Input: part model. Units: mm. Frame: model coordinates. Face numbers are marked on the shaded views. A direction names the side the tool comes from. Round coordinates to 2 decimals unless told otherwise and drop trailing zeros. Order: outer loops, then holes, each group sorted by start corner. A loop starts at its lowest first (then second) coordinate and runs counter-clockwise, first axis right, second up. Notation, with made-up numbers: (13, 19) -> (20, 19) arc R22 cw to (20, 56) -> close; hole circle Ø8 at (13, -39). An arc over 180 degrees is marked (long way). Use a Markdown table: item, result.
from build123d import *

# Parameters (mm, degrees)
BOSS_EXTRUDE1_DEPTH         = 2
SKETCH5_R                   = 4
SKETCH5_R_2                 = 1.998542518
BOSS_EXTRUDE2_DEPTH         = 3
SKETCH8_R                   = 1.5
CUT_EXTRUDE2_DEPTH          = 6
SKETCH9_R                   = 3.6
SKETCH9_R_2                 = 3
BOSS_EXTRUDE3_DEPTH         = 0.85
SKETCH10_R                  = 0.75
CUT_EXTRUDE3_DEPTH          = 2
LPATTERN1_COUNT             = 4
LPATTERN1_PITCH             = 3.5
CIRPATTERN1_COUNT           = 4
CIRPATTERN1_COPY_1_SKETCH_R = 0.75
CIRPATTERN1_COPY_1_DEPTH    = 2
CIRPATTERN1_COPY_2_SKETCH_R = 0.75
CIRPATTERN1_COPY_2_DEPTH    = 2
CIRPATTERN1_COPY_3_SKETCH_R = 0.75
CIRPATTERN1_COPY_3_DEPTH    = 2
CIRPATTERN1_COPY_4_SKETCH_R = 0.75
CIRPATTERN1_COPY_4_DEPTH    = 2
CIRPATTERN1_COPY_5_SKETCH_R = 0.75
CIRPATTERN1_COPY_5_DEPTH    = 2
CIRPATTERN1_COPY_6_SKETCH_R = 0.75
CIRPATTERN1_COPY_6_DEPTH    = 2
CIRPATTERN1_COPY_7_SKETCH_R = 0.75
CIRPATTERN1_COPY_7_DEPTH    = 2
CIRPATTERN1_COPY_8_SKETCH_R = 0.75
CIRPATTERN1_COPY_8_DEPTH    = 2
CIRPATTERN1_COPY_9_SKETCH_R = 0.75
CIRPATTERN1_COPY_9_DEPTH    = 2


with BuildPart() as part:
    # Sketch1 → Boss-Extrude1 (new body)
    with BuildSketch(Plane(origin=(0, 0, 0), x_dir=(1, 0, 0), z_dir=(0, 1, 0))):
        with BuildLine():
            Line((11.195476756, 1.969359322), (4.786657556, -6.592741724))
            ThreePointArc((4.786657556, -6.592741724), (3.929987754, -8.118293207), (4.786657556, -9.643844691))
            Line((4.786657556, -9.643844691), (11.195476756, -18.205945736))
            ThreePointArc((11.195476756, -18.205945736), (10.933214648, -21.871520101), (7.267640283, -22.133782209))
            Line((7.267640283, -22.133782209), (-1.294460762, -15.724963009))
            ThreePointArc((-1.294460762, -15.724963009), (-2.820012246, -14.868293207), (-4.34556373, -15.724963009))
            Line((-4.34556373, -15.724963009), (-12.907664775, -22.133782209))
            ThreePointArc((-12.907664775, -22.133782209), (-16.57323914, -21.871520101), (-16.835501248, -18.205945736))
            Line((-16.835501248, -18.205945736), (-10.426682048, -9.643844691))
            ThreePointArc((-10.426682048, -9.643844691), (-9.570012246, -8.118293207), (-10.426682048, -6.592741724))
            Line((-10.426682048, -6.592741724), (-16.835501248, 1.969359322))
            ThreePointArc((-16.835501248, 1.969359322), (-16.57323914, 5.634933687), (-12.907664775, 5.897195795))
            Line((-12.907664775, 5.897195795), (-4.34556373, -0.511623405))
            ThreePointArc((-4.34556373, -0.511623405), (-2.820012246, -1.368293207), (-1.294460762, -0.511623405))
            Line((-1.294460762, -0.511623405), (7.267640283, 5.897195795))
            ThreePointArc((7.267640283, 5.897195795), (10.933214648, 5.634933687), (11.195476756, 1.969359322))
        make_face()
    extrude(amount=BOSS_EXTRUDE1_DEPTH)

    # Sketch5 → Boss-Extrude2 (add)
    with BuildSketch(Plane(origin=(0, 2, 0), x_dir=(1, 0, 0), z_dir=(0, 1, 0))):
        with Locations((-2.820012246, -8.118293207)):
            Circle(SKETCH5_R)
        with Locations((-2.820012246, -8.118293207)):
            Circle(SKETCH5_R_2, mode=Mode.SUBTRACT)
    extrude(amount=BOSS_EXTRUDE2_DEPTH)

    # Sketch8 → Cut-Extrude2 (cut, through all)
    with BuildSketch(Plane.XZ):
        with Locations((-2.820012246, 8.118293207)):
            Circle(SKETCH8_R)
    extrude(amount=-CUT_EXTRUDE2_DEPTH, mode=Mode.SUBTRACT)

    # Sketch9 → Boss-Extrude3 (add)
    with BuildSketch(Plane.XZ):
        with Locations((-2.820012246, 8.118293207)):
            Circle(SKETCH9_R)
        with Locations((-2.820012246, 8.118293207)):
            Circle(SKETCH9_R_2, mode=Mode.SUBTRACT)
    extrude(amount=BOSS_EXTRUDE3_DEPTH)

    # Sketch10 → Cut-Extrude3 (cut)
    with BuildSketch(Plane.XZ):
        with Locations((9.519001086, -4.220720125)):
            Circle(SKETCH10_R)
    cut_extrude3 = extrude(amount=-CUT_EXTRUDE3_DEPTH, mode=Mode.SUBTRACT)

    # LPattern1: Cut-Extrude3 ×4
    with Locations(*[Vector(-0.707106781, 0, 0.707106781) * (i * LPATTERN1_PITCH) for i in range(1, LPATTERN1_COUNT)]):
        add(cut_extrude3, mode=Mode.SUBTRACT)

    # CirPattern1: Cut-Extrude3 ×4 about axis
    cirpattern1_axis = Axis((-2.820012246, 0, 8.118293207), (0, 1, 0))
    for i in range(1, CIRPATTERN1_COUNT):
        add(cut_extrude3.rotate(cirpattern1_axis, i * 360 / CIRPATTERN1_COUNT), mode=Mode.SUBTRACT)

    # CirPattern1 copy 1 sketch → CirPattern1 copy 1 (cut)
    with BuildSketch(Plane(origin=(-8.463431719, 0, 7.773154695), x_dir=(0, 0, -1), z_dir=(0, -1, 0))):
        with Locations((9.519001086, -4.220720125)):
            Circle(CIRPATTERN1_COPY_1_SKETCH_R)
    extrude(amount=-CIRPATTERN1_COPY_1_DEPTH, mode=Mode.SUBTRACT)

    # CirPattern1 copy 2 sketch → CirPattern1 copy 2 (cut)
    with BuildSketch(Plane(origin=(-3.165150758, 0, 13.76171268), x_dir=(-1, 0, 0), z_dir=(0, -1, 0))):
        with Locations((9.519001086, -4.220720125)):
            Circle(CIRPATTERN1_COPY_2_SKETCH_R)
    extrude(amount=-CIRPATTERN1_COPY_2_DEPTH, mode=Mode.SUBTRACT)

    # CirPattern1 copy 3 sketch → CirPattern1 copy 3 (cut)
    with BuildSketch(Plane(origin=(2.823407227, 0, 8.463431719), x_dir=(0, 0, 1), z_dir=(0, -1, 0))):
        with Locations((9.519001086, -4.220720125)):
            Circle(CIRPATTERN1_COPY_3_SKETCH_R)
    extrude(amount=-CIRPATTERN1_COPY_3_DEPTH, mode=Mode.SUBTRACT)

    # CirPattern1 copy 4 sketch → CirPattern1 copy 4 (cut)
    with BuildSketch(Plane(origin=(-5.988557985, 0, 10.248028429), x_dir=(0, 0, -1), z_dir=(0, -1, 0))):
        with Locations((9.519001086, -4.220720125)):
            Circle(CIRPATTERN1_COPY_4_SKETCH_R)
    extrude(amount=-CIRPATTERN1_COPY_4_DEPTH, mode=Mode.SUBTRACT)

    # CirPattern1 copy 5 sketch → CirPattern1 copy 5 (cut)
    with BuildSketch(Plane(origin=(-0.690277024, 0, 11.286838946), x_dir=(-1, 0, 0), z_dir=(0, -1, 0))):
        with Locations((9.519001086, -4.220720125)):
            Circle(CIRPATTERN1_COPY_5_SKETCH_R)
    extrude(amount=-CIRPATTERN1_COPY_5_DEPTH, mode=Mode.SUBTRACT)

    # CirPattern1 copy 6 sketch → CirPattern1 copy 6 (cut)
    with BuildSketch(Plane(origin=(0.348533493, 0, 5.988557985), x_dir=(0, 0, 1), z_dir=(0, -1, 0))):
        with Locations((9.519001086, -4.220720125)):
            Circle(CIRPATTERN1_COPY_6_SKETCH_R)
    extrude(amount=-CIRPATTERN1_COPY_6_DEPTH, mode=Mode.SUBTRACT)

    # CirPattern1 copy 7 sketch → CirPattern1 copy 7 (cut)
    with BuildSketch(Plane(origin=(-3.513684251, 0, 12.722902164), x_dir=(0, 0, -1), z_dir=(0, -1, 0))):
        with Locations((9.519001086, -4.220720125)):
            Circle(CIRPATTERN1_COPY_7_SKETCH_R)
    extrude(amount=-CIRPATTERN1_COPY_7_DEPTH, mode=Mode.SUBTRACT)

    # CirPattern1 copy 8 sketch → CirPattern1 copy 8 (cut)
    with BuildSketch(Plane(origin=(1.78459671, 0, 8.811965212), x_dir=(-1, 0, 0), z_dir=(0, -1, 0))):
        with Locations((9.519001086, -4.220720125)):
            Circle(CIRPATTERN1_COPY_8_SKETCH_R)
    extrude(amount=-CIRPATTERN1_COPY_8_DEPTH, mode=Mode.SUBTRACT)

    # CirPattern1 copy 9 sketch → CirPattern1 copy 9 (cut)
    with BuildSketch(Plane(origin=(-2.126340241, 0, 3.513684251), x_dir=(0, 0, 1), z_dir=(0, -1, 0))):
        with Locations((9.519001086, -4.220720125)):
            Circle(CIRPATTERN1_COPY_9_SKETCH_R)
    extrude(amount=-CIRPATTERN1_COPY_9_DEPTH, mode=Mode.SUBTRACT)


solid = part.part
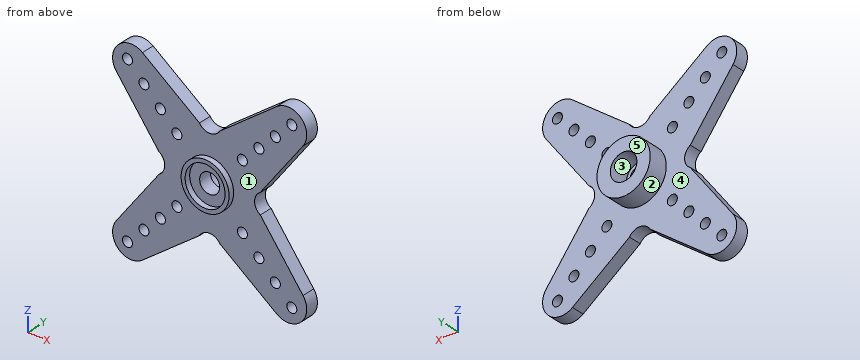
1) Cut plane A-A on z = -3. Return loops of the section in (x, y), and give its area (3 significant figures).
Results found:
| item | result |
|---|---|
| outline | (-17.32, 0) -> (-9.04, 0) -> (-9.04, 2) -> (-17.32, 2) -> close; (3.4, 0) -> (11.68, 0) -> (11.68, 2) -> (3.4, 2) -> close |
| area | 33.1 mm² |
2) Cut plane B-B on y = 4.4. Return loops of the section in (x, z), and give its area (3 significant figures).
Results found:
| item | result |
|---|---|
| outline | circle Ø8 at (-2.82, 8.12); hole circle Ø4 at (-2.82, 8.12) |
| area | 37.7 mm² |
3) Cut plane C-C on z = 7. Return loops of the section in (x, y).
Results found:
| item | result |
|---|---|
| outline | (-9.96, 0) -> (-6.24, 0) -> (-6.24, -0.85) -> (-5.6, -0.85) -> (-5.6, 0) -> (-3.82, 0) -> (-3.82, 2) -> (-4.48, 2) -> (-4.48, 5) -> (-6.66, 5) -> (-6.66, 2) -> (-9.96, 2) -> close; (-1.82, 0) -> (-0.04, 0) -> (-0.04, -0.85) -> (0.6, -0.85) -> (0.6, 0) -> (4.32, 0) -> (4.32, 2) -> (1.02, 2) -> (1.02, 5) -> (-1.16, 5) -> (-1.16, 2) -> (-1.82, 2) -> close |
4) Pull-direction query (Z, two-part tool) for the marked faces 1, 2 and 3; classes: +Z half, -Z half, draft (parallel to the pull), parting line (faces both ways), or undercut.
Results found:
| item | result |
|---|---|
| face 1 | draft |
| face 2 | parting line |
| face 3 | undercut |
5) Pin query (flat end, axial travel): pin 1 Ø3 at (x, y) = (-14, 0.5) entering from -Z; pin 2 Ø10 at (x, z) = (-7.5, 18.5) entering from -Y; pin 3 Ø2.5 at (x, z) = (-15.16, 20.46) entering from +Y. Return the tip coordinate at first contact, or that it passes through.
Results found:
| item | result |
|---|---|
| pin 1 | stops at z = -6.46 |
| pin 2 | stops at y = 0 |
| pin 3 | stops at y = 2 |
6) Line query: L1, parallel to X at y = 2.25, z = 8; L2, parallel to X at y = 1.6, z = 20; L3, parallel to Z at x = -7.25, y = 0.2. Output: solid intervals per line, ascending. Write a range as [from, to].
Results found:
| item | result |
|---|---|
| L1 | x = [-6.82, -4.82], [-0.82, 1.18] |
| L2 | x = [-17.39, -15.75], [-14.56, -10.06], [4.42, 8.92], [10.11, 11.75] |
| L3 | z = [-1.66, 2.63], [3.78, 12.46], [13.61, 17.9] |
7) Set-up query: the marked faces 4 and 5. Return all of +Z, -Z, +X, -X, +Y, -Y with unobstructed straight access to the full face (end or side cutting, diameter ignored); none if empty.
Results found:
| item | result |
|---|---|
| face 4 | +Y |
| face 5 | +Z, -Z, +X, -X, +Y |
